Can you work these out from the model? Positions are in its coordinate system, mm. A direction names the side the tool comes from. Give positions to 0.01 mm unless a question says otherwise; leave off trailing zeros. Loops run counter-clockwise (first coordinate to the right, second up) from the corner with the lowest first, then second, coordinate; pieces in that order, holes last. Notation, with made-up numbers: M 2,-14 L 15,-14 A3 ccw 15,-9 Z; hole C 7.25,-34 d7. An arc over 180 degrees is marked long. Put each result on its own line as item: value. Start each with the question number.
1) Imagine slicing it at D-D (y = -10.5). Write out the boundary of the cut face in (x, z), then the cut area to 3 significant figures.
2) Imagine slicing it at B-B (y = -17.78). Write out the boundary of the cut face in (x, z).
3) Please list where these lines run through material, in increasing order: line 1 along X through (y, z) = (-6.5, 5.75); line 2 along Y through (x, z) = (4, 7); line 3 along Z through (x, y) = (-15.65, -17.78). Write a range as from..to.
4) Imagine slicing it at A-A (z = 4). Write out the boundary of the cut face in (x, y).
5) Imagine slicing it at C-C (z = 10.25). Write out the boundary of the cut face in (x, y) (1 decimal).
6) For faces 5 (the cylindrical face through (-11.089, -0.986, 2.096)), 6 (the flat face through (16.16, -11, 5)), 7 (the cylindrical face through (13.779, -2.362, 6.042)), which set-ups out of +Z, -Z, +X, -X, +Y, -Y let a thin tool reach every point of the face, with its end or its side?
7) If we mould it in two halves opening along Z, with no side actions, what happens to faces 1 (the cylindrical face through (-15.174, -22.286, 7.191)), 2 (the flat face through (-12.192, -1, 6)), 3 (the cylindrical face through (-13.798, -2.382, 6.042)), 4 (the cylindrical face through (15.174, -16.688, 5.713))? For each: +Z half, -Z half, draft (parallel to the pull), parting line (faces both ways), or undercut.
8) For P1, Ø2, axis at y = -1, z = 6.5, coming from the +X side; P2, Ø1.5, axis at x = -9, z = 7, coming from the +Y side; P3, Ø6, axis at x = -1.5, z = 4.5, coming from the -Y side; P4, Ø0.6, axis at y = -1, z = 5.5, coming from the -X side, each with a flat end and sliding along its axis, tell me the tip position at first contact or that it passes through.
from build123d import *

# Parameters (mm, degrees)
F1_DEPTH      = 12.7
F3_DEPTH      = 16.1615
F3_DEPTH_BACK = 16.1615
F4_R          = 2.032
F5_DEPTH      = 32.322
F5_DEPTH_BACK = 60
F6_R          = 2.54
F8_DEPTH      = 22.861


# Not quite as in the source:
# - an extrude ends at something that could not be found from the text; its depth is read off the source's solid
# - a feature names something its author has since deleted; it is built from what else it names


with BuildPart() as f1:
    # F0 (on Top) → F1 (new body)
    with BuildSketch(Plane.XY):
        with BuildLine():
            Line((13.6205, 0), (0, 0))
            Line((0, 0), (-13.6205, 0))
            ThreePointArc((-13.6205, 0), (-15.4165512242, -0.7439487758), (-16.1605, -2.54))
            Line((-16.1605, -2.54), (-16.1605, -22.86))
            Line((-16.1605, -22.86), (-14.1605, -22.86))
            Line((-14.1605, -22.86), (-14.1605, -3.27))
            ThreePointArc((-14.1605, -3.27), (-13.7885256121, -2.3719743879), (-12.8905, -2))
            Line((-12.8905, -2), (0, -2))
            Line((0, -2), (12.8905, -2))
            ThreePointArc((12.8905, -2), (13.7885256121, -2.3719743879), (14.1605, -3.27))
            Line((14.1605, -3.27), (14.1605, -22.86))
            Line((14.1605, -22.86), (16.1605, -22.86))
            Line((16.1605, -22.86), (16.1605, -2.54))
            ThreePointArc((16.1605, -2.54), (15.4165512242, -0.7439487758), (13.6205, 0))
        make_face()
    extrude(amount=F1_DEPTH)

    # F2 (on Right) → F3 (cut, two sides)
    with BuildSketch(Plane.YZ) as f3_sk:
        Polygon((0, 12.7), (-2.54, 12.7), (-22.86, 12.7), (-22.86, 7.62), align=None)
    extrude(amount=-F3_DEPTH, mode=Mode.SUBTRACT)
    extrude(f3_sk.sketch, amount=F3_DEPTH_BACK, mode=Mode.SUBTRACT)

    # F4 (on face) → F5 (cut, two sides)
    with BuildSketch(Plane.YZ.offset(16.1605)) as f5_sk:
        with Locations((-17.78, 4)):
            Circle(F4_R)
    extrude(amount=-F5_DEPTH, mode=Mode.SUBTRACT)
    extrude(f5_sk.sketch, amount=F5_DEPTH_BACK, mode=Mode.SUBTRACT)

    # F6
    f6_edges = [f1.edges().sort_by_distance(p)[0] for p in [
        (15.1605, -22.86, 7.62),
        (-15.1605, -22.86, 7.62),
        (-15.1605, -22.86, 0),
        (15.1605, -22.86, 0),
    ]]
    fillet(f6_edges, radius=F6_R)

    # F7 (on face) → F8 (cut, through all)
    with BuildSketch(Plane(origin=(0, 0, 0), x_dir=(-1, 0, 0), z_dir=(0, 1, 0))):
        with BuildLine():
            Line((-10.033, 3.175), (-10.033, 9.525))
            ThreePointArc((-10.033, 9.525), (-11.1125, 10.6045), (-12.192, 9.525))
            Line((-12.192, 9.525), (-12.192, 3.175))
            ThreePointArc((-12.192, 3.175), (-11.1125, 2.0955), (-10.033, 3.175))
        make_face()
        with BuildLine():
            ThreePointArc((10.033, 3.175), (11.1125, 2.0955), (12.192, 3.175))
            Line((12.192, 3.175), (12.192, 9.525))
            ThreePointArc((12.192, 9.525), (11.1125, 10.6045), (10.033, 9.525))
            Line((10.033, 9.525), (10.033, 3.175))
        make_face()
    extrude(amount=-F8_DEPTH, mode=Mode.SUBTRACT)


solid = f1.part
Recorded:
1. outline: M -16.16,0 L -14.16,0 L -14.16,10.37 L -16.16,10.37 Z; M 14.16,0 L 16.16,0 L 16.16,10.37 L 14.16,10.37 Z
1. area: 41.5 mm²
2. outline: M -16.16,0 L -14.16,0 L -14.16,1.97 L -16.16,1.97 Z; M -16.16,6.03 L -14.16,6.03 L -14.16,8.75 L -16.16,8.75 Z; M 14.16,0 L 16.16,0 L 16.16,1.97 L 14.16,1.97 Z; M 14.16,6.03 L 16.16,6.03 L 16.16,8.75 L 14.16,8.75 Z
3. line 1: -16.16..-14.16, 14.16..16.16
3. line 2: -2..0
3. line 3: 0..1.97, 6.03..8.75
4. outline: M -16.16,-22.86 L -14.16,-22.86 L -14.16,-19.81 L -16.16,-19.81 Z; M -16.16,-15.75 L -14.16,-15.75 L -14.16,-3.27 A1.27 cw -12.89,-2 L -12.19,-2 L -12.19,0 L -13.62,0 A2.54 ccw -16.16,-2.54 Z; M -10.03,-2 L 10.03,-2 L 10.03,0 L -10.03,0 Z; M 12.19,-2 L 12.89,-2 A1.27 cw 14.16,-3.27 L 14.16,-15.75 L 16.16,-15.75 L 16.16,-2.54 A2.54 ccw 13.62,0 L 12.19,0 Z; M 14.16,-22.86 L 16.16,-22.86 L 16.16,-19.81 L 14.16,-19.81 Z
5. outline: M -16.2,-11 L -14.2,-11 L -14.2,-3.3 A1.3 cw -12.9,-2 L -11.9,-2 L -11.9,0 L -13.6,0 A2.5 ccw -16.2,-2.5 Z; M -10.3,-2 L 10.3,-2 L 10.3,0 L -10.3,0 Z; M 11.9,-2 L 12.9,-2 A1.3 cw 14.2,-3.3 L 14.2,-11 L 16.2,-11 L 16.2,-2.5 A2.5 ccw 13.6,0 L 11.9,0 Z
6. face 5: +Y, -Y
6. face 6: +Z, -Z, +X, +Y, -Y
6. face 7: +Z, -Z, -Y
7. face 1: +Z half
7. face 2: undercut
7. face 3: draft
7. face 4: undercut
8. P1: x = 16.1
8. P2: y = 0
8. P3: y = -2
8. P4: x = -15.84
